from build123d import *

# Parameters (mm, degrees)
F0_R     = 1.5
F1_DEPTH = 1
F2_R     = 3.99999
F3_R     = 0.5
F4_DEPTH = 25


# Not quite as in the source:
# - a fillet or chamfer is up to 0.001 mm smaller than in the source, because OpenCascade refuses the exact size


with BuildPart() as f1:
    # F0 (on Right) → F1 (new body)
    with BuildSketch(Plane.YZ):
        Polygon((0, 30), (0, 0), (7, 0), (7, -1.5), (15, -1.5), (15, 0), (20, 0), (20, 15.5), (24, 15.5), (24, 30), (15, 30), (15, 31.5), (7, 31.5), (7, 30), align=None)
        with Locations((12.5, 15)):
            Circle(F0_R, mode=Mode.SUBTRACT)
    extrude(amount=F1_DEPTH)

    # F2 (radius 4 in the source; OpenCascade refuses exactly that, so slightly less here)
    f2_edges = [f1.edges().sort_by_distance(p)[0] for p in [
        (0.5, 20, 15.5),
    ]]
    fillet(f2_edges, radius=F2_R)

    # F3 (on face) → F4 (cut)
    with BuildSketch(Plane.YZ.offset(1)):
        with Locations((6.5, 30)):
            Circle(F3_R)
        with Locations((15.5, 30)):
            Circle(F3_R)
        with Locations((6.5, 0)):
            Circle(F3_R)
        with Locations((15.5, 0)):
            Circle(F3_R)
    extrude(amount=-F4_DEPTH, mode=Mode.SUBTRACT)


solid = f1.part
Design review of the part built by this model. Coordinates are the model's own, in mm. A direction names the side the tool comes from. Coordinates: 2 decimals unless noted, no trailing zeros. Write each loop counter-clockwise with the first axis right and the second up, starting at its lowest first coordinate (ties: lowest second). Pieces come first, ordered by that corner, then holes. Notation, with made-up numbers: (3.25, 53) - (35.25, 53) arc R29 cw to (35.25, 82) - close; hole circle Ø1 at (-35, 3.25). An arc over 180 degrees is marked (long way). Use one line per item in the form item = value.
Q1. Insertion check: pin 1 Ø0.5 at (x, y) = (0.5, 19) entering from +Z; pin 2 Ø0.5 at (x, z) = (0.5, -0.5) entering from +Y; pin 3 Ø0.5 at (x, z) = (0.5, 30.5) entering from -Y. Each pin has a flat end and moves straight along its axis. Give the tip position at first contact, or say it passes through.
Taken from the geometry:
pin_1 = 30
pin_2 = 15
pin_3 = 7
Q2. Consider section A-A (y = 12.5). Write out the cut boundary in (x, z), plus the area to 3 significant figures.
Taken from the geometry:
outline = (0, -1.5) - (1, -1.5) - (1, 13.5) - (0, 13.5) - close; (0, 16.5) - (1, 16.5) - (1, 31.5) - (0, 31.5) - close
area = 30.0 mm^2
Q3. The part is to be moulded in two halves that separate along Y. For faces 6 (the cylindrical face through (0.49, 11.39, 16.01)), 7 (the flat face through (0.5, 10.9, -1.5)), 8 (the cylindrical face through (0.507, 21.141, 14.297)), say which applies: +Y half, -Y half, draft (parallel to the pull), parting line (faces both ways), or undercut.
Taken from the geometry:
face_6 = undercut
face_7 = draft
face_8 = +Y half
Q4. Machinability: for faces 1 (the flat face through (0.5, 7, -0.7)), 2 (the flat face through (0.5, 7, 30.8)), 3 (the cylindrical face through (0.5, 6.5, 29.5)), 4 (the flat face through (0.5, 20.1, 30)), 5 (the flat face through (0.5, 18, 0)), which of the approach directions +Z, -Z, +X, -X, +Y, -Y give a long, thin tool a straight path to every point of the face, cutting with its end or side? Answer none if there is none.
Taken from the geometry:
face_1 = -Z, +X, -X, -Y
face_2 = +Z, +X, -X, -Y
face_3 = +Z, +X, -X
face_4 = +Z, +X, -X, +Y
face_5 = -Z, +X, -X, +Y
Q5. Consider section D-D (z = 11). Write out the cut boundary in (x, y), plus the area to 3 significant figures.
Taken from the geometry:
outline = (0, 0) - (1, 0) - (1, 20) - (0, 20) - close
area = 20.0 mm^2
Q6. Consider section C-C (z = 15). Write out the cut boundary in (x, y).
Taken from the geometry:
outline = (0, 0) - (1, 0) - (1, 11) - (0, 11) - close; (0, 14) - (1, 14) - (1, 22.06) - (0, 22.06) - close
Q7. For probe 1 along Z at (x, y) = (0.6, 12.5); probe 2 along Z at (x, y) = (0.8, 1); probe 3 along Z at (x, y) = (0.7, 12), list the stretches that pass through material, from the lowest coordinate up.
Taken from the geometry:
probe_1 = -1.5 to 13.5, 16.5 to 31.5
probe_2 = 0 to 30
probe_3 = -1.5 to 13.59, 16.41 to 31.5
